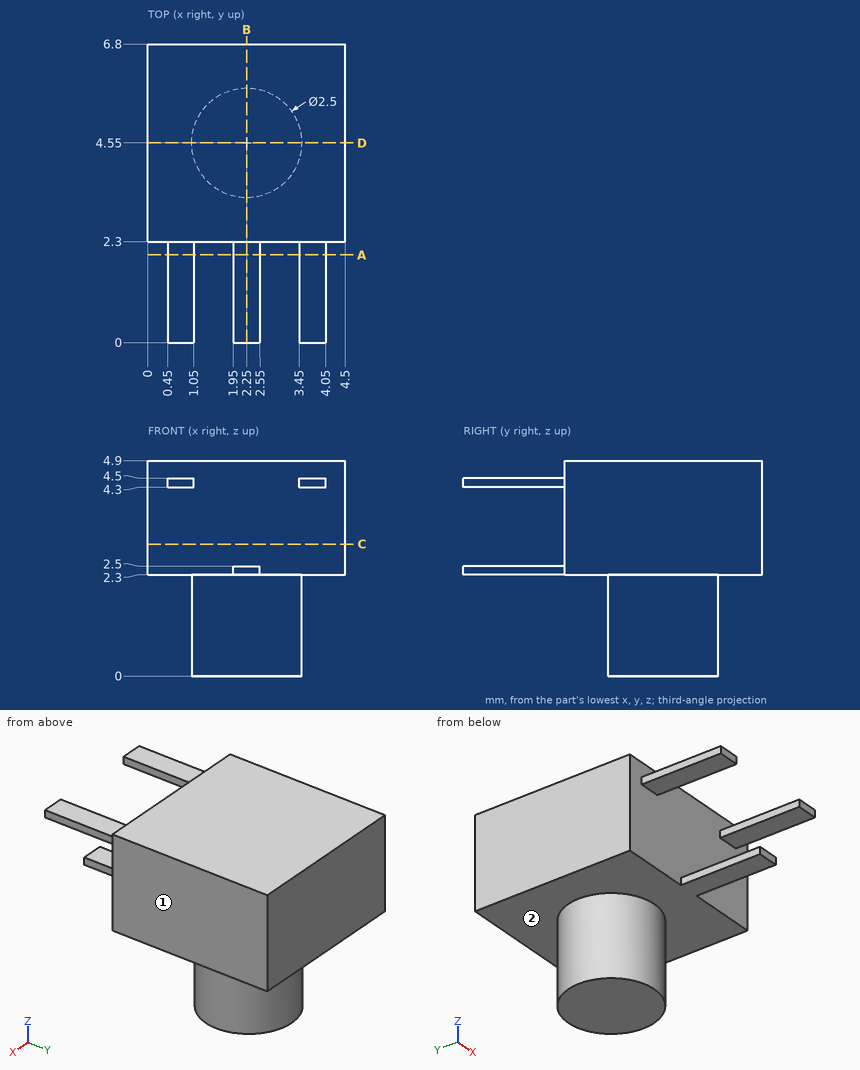
For this review, use the dimensioned drawing (mm, ordinates from the lowest corner) and the shaded views. A direction names the side the tool comes from. Give positions to 0.01 mm unless a question says otherwise; leave off trailing zeros. Write each loop counter-clockwise with the first axis right and the second up, starting at its lowest first coordinate (ties: lowest second). Pieces come first, ordered by that corner, then holes. Notation, with made-up numbers: M 37,33 L 87,33 A32 cw 87,70 Z; hole C 5.5,-29.5 d10. An arc over 180 degrees is marked long. Write item = value, one per line. Start each with the question number.
Q1. We need section B-B (x = 2.25). State the section outline as (y, z) points, plus the area to 3 significant figures.
Q2. We need section C-C (z = 3). State the section outline as (x, y) points, plus the area to 4 significant figures.
Q3. For line 1 (X direction, y = 1, z = 2.35); line 2 (X direction, y = 4.5, z = 0.75); line 3 (Y direction, x = 3.95, z = 4.25), list the stretches that pass through material, from the lowest coordinate up.
Q4. Clearance check with flat-ended pins moving along their axes: pin 1 (0.5 mm diameter, centred on x = 0.5, y = 1.5, fed in from -Z); pin 2 (0.7 mm diameter, centred on x = 0.5, y = 1, fed in from +Z); pin 3 (0.5 mm diameter, centred on x = 2.5, y = 1, fed in from +Z). State where each tip first meets the part, or that it passes through.
Q5. We need section A-A (y = 2). State the section outline as (x, z) points.
Q6. Machinability: for the marked faces 1 and 2, which of the approach directions +Z, -Z, +X, -X, +Y, -Y give a long, thin tool a straight path to every point of the face, cutting with its end or side? Answer none if there is none.
Q7. We need section D-D (y = 4.55). State the section outline as (x, z) points.
Result set:
q1.outline = M 0,2.3 L 3.3,2.3 L 3.3,0 L 5.8,0 L 5.8,2.3 L 6.8,2.3 L 6.8,4.9 L 2.3,4.9 L 2.3,2.5 L 0,2.5 Z
q1.area = 17.9 mm2
q2.outline = M 0,2.3 L 4.5,2.3 L 4.5,6.8 L 0,6.8 Z
q2.area = 20.25 mm2
q3.line_1 = 1.95 to 2.55
q3.line_2 = 1 to 3.5
q3.line_3 = 2.3 to 6.8
q4.pin_1 = 4.3
q4.pin_2 = 4.5
q4.pin_3 = 2.5
q5.outline = M 0.45,4.3 L 1.05,4.3 L 1.05,4.5 L 0.45,4.5 Z; M 1.95,2.3 L 2.55,2.3 L 2.55,2.5 L 1.95,2.5 Z; M 3.45,4.3 L 4.05,4.3 L 4.05,4.5 L 3.45,4.5 Z
q6.face_1 = +Z, -Z, +X, +Y, -Y
q6.face_2 = -Z
q7.outline = M 0,2.3 L 1,2.3 L 1,0 L 3.5,0 L 3.5,2.3 L 4.5,2.3 L 4.5,4.9 L 0,4.9 Z
